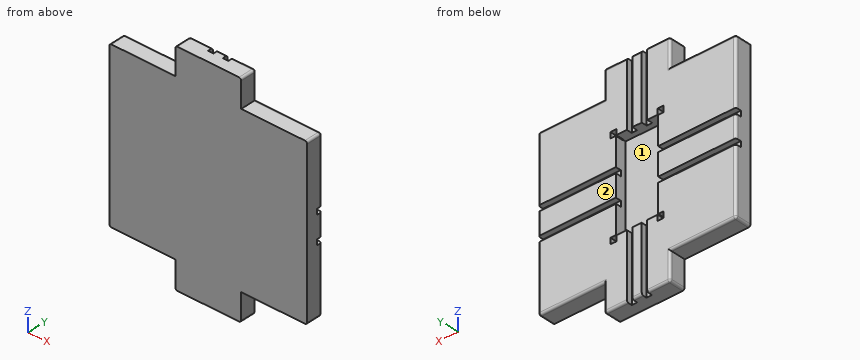
```python
from build123d import *

# Parameters (mm, degrees)
SKETCH1_W                                  = 180
SKETCH1_H                                  = 150
BOSS_EXTRUDE1_DEPTH                        = 15
SKETCH7_W                                  = 60
SKETCH7_H                                  = 25
BOSS_EXTRUDE6_DEPTH                        = 15
FILLET1_R                                  = 2
SKETCH2_W                                  = 38.5
SKETCH2_H                                  = 82
CUT_EXTRUDE1_DEPTH                         = 10
CUT_EXTRUDE3_DEPTH                         = 5
SKETCH11_W                                 = 5.5
SKETCH11_H                                 = 5.5
CUT_EXTRUDE6_DEPTH                         = 7
MIRROR3_AT_THE_SECOND_PLANE_COPY_1_SKETC_W = 5.5
MIRROR3_AT_THE_SECOND_PLANE_COPY_1_SKETC_H = 5.5
MIRROR3_AT_THE_SECOND_PLANE_COPY_1_DEPTH   = 7
MIRROR4_AT_THE_SECOND_PLANE_COPY_1_DEPTH   = 5


with BuildPart() as part:
    # Sketch1 → Boss-Extrude1 (new body)
    with BuildSketch(Plane(origin=(0, 0, 0), x_dir=(1, 0, 0), z_dir=(0, 1, 0))):
        Rectangle(SKETCH1_W, SKETCH1_H)
    extrude(amount=BOSS_EXTRUDE1_DEPTH)

    # Sketch7 → Boss-Extrude6 (add)
    with BuildSketch(Plane(origin=(0, 0, 0), x_dir=(1, 0, 0), z_dir=(0, 1, 0))):
        with Locations((0, -87.5)):
            Rectangle(SKETCH7_W, SKETCH7_H)
        with Locations((0, 87.5)):
            Rectangle(SKETCH7_W, SKETCH7_H)
    extrude(amount=BOSS_EXTRUDE6_DEPTH)

    # Fillet1
    fillet1_edges = [part.edges().sort_by_distance(p)[0] for p in [
        (-90, 15, 0),
        (60, 15, 75),
        (-60, 15, 75),
        (-30, 7.5, 100),
        (30, 7.5, 100),
        (-30, 15, 87.5),
        (0, 15, 100),
        (30, 15, 87.5),
        (-60, 15, -75),
        (0, 15, -100),
        (30, 7.5, -100),
        (-30, 15, -87.5),
        (-30, 7.5, -100),
        (30, 15, -87.5),
        (90, 15, 0),
        (90, 7.5, 75),
        (-90, 7.5, 75),
        (-90, 7.5, -75),
        (90, 7.5, -75),
        (60, 15, -75),
    ]]
    fillet(fillet1_edges, radius=FILLET1_R)

    # Sketch2 → Cut-Extrude1 (cut)
    with BuildSketch(Plane(origin=(0, 15, 0), x_dir=(1, 0, 0), z_dir=(0, 1, 0))):
        Rectangle(SKETCH2_W, SKETCH2_H)
    extrude(amount=-CUT_EXTRUDE1_DEPTH, mode=Mode.SUBTRACT)

    # Sketch10 → Cut-Extrude3 (cut)
    with BuildSketch(Plane(origin=(0, 15, 0), x_dir=(1, 0, 0), z_dir=(0, 1, 0))):
        Polygon((-9.25, -40.5), (-9.25, -33.162899401), (-4.25, -33.162899401), (-4.25, -40.5), (-4.25, -105.687952047), (-9.25, -105.687952047), align=None)
        Polygon((-99.022946063, 15), (-19.25, 15), (-11.555108838, 15), (-11.555108838, 10), (-19.25, 10), (-99.022946063, 10), align=None)
    cut_extrude3 = extrude(amount=-CUT_EXTRUDE3_DEPTH, mode=Mode.SUBTRACT)

    # Sketch11 → Cut-Extrude6 (cut)
    with BuildSketch(Plane(origin=(0, 15, 0), x_dir=(1, 0, 0), z_dir=(0, 1, 0))):
        with Locations((-21.549732367, 43.299732367)):
            Rectangle(SKETCH11_W, SKETCH11_H)
    cut_extrude6 = extrude(amount=-CUT_EXTRUDE6_DEPTH, mode=Mode.SUBTRACT)

    # Mirror3: Cut-Extrude6 across plane
    add(cut_extrude6.mirror(Plane(origin=(0, 0, 0), x_dir=(0, 0, 1), z_dir=(1, 0, 0))), mode=Mode.SUBTRACT)

    # Mirror3 at the second plane: Cut-Extrude6 across plane
    add(cut_extrude6.mirror(Plane.XY), mode=Mode.SUBTRACT)

    # Mirror3 at the second plane copy 1 sketc → Mirror3 at the second plane copy 1 (cut)
    with BuildSketch(Plane(origin=(0, 15, 0), x_dir=(-1, 0, 0), z_dir=(0, 1, 0))):
        with Locations((-21.549732367, 43.299732367)):
            Rectangle(MIRROR3_AT_THE_SECOND_PLANE_COPY_1_SKETC_W, MIRROR3_AT_THE_SECOND_PLANE_COPY_1_SKETC_H)
    extrude(amount=-MIRROR3_AT_THE_SECOND_PLANE_COPY_1_DEPTH, mode=Mode.SUBTRACT)

    # Mirror4: Cut-Extrude3 across plane
    add(cut_extrude3.mirror(Plane(origin=(0, 0, 0), x_dir=(0, 0, 1), z_dir=(1, 0, 0))), mode=Mode.SUBTRACT)

    # Mirror4 at the second plane: Cut-Extrude3 across plane
    add(cut_extrude3.mirror(Plane.XY), mode=Mode.SUBTRACT)

    # Mirror4 at the second plane copy 1 sketc → Mirror4 at the second plane copy 1 (cut)
    with BuildSketch(Plane(origin=(0, 15, 0), x_dir=(-1, 0, 0), z_dir=(0, 1, 0))):
        Polygon((-9.25, -40.5), (-9.25, -33.162899401), (-4.25, -33.162899401), (-4.25, -40.5), (-4.25, -105.687952047), (-9.25, -105.687952047), align=None)
        Polygon((-99.022946063, 15), (-19.25, 15), (-11.555108838, 15), (-11.555108838, 10), (-19.25, 10), (-99.022946063, 10), align=None)
    extrude(amount=-MIRROR4_AT_THE_SECOND_PLANE_COPY_1_DEPTH, mode=Mode.SUBTRACT)


solid = part.part
```
For this review, take the finished solid that the model builds, in its own axes (mm). Face numbers are marked on the shaded views. Coordinates: 2 decimals unless noted, no trailing zeros. Write each loop counter-clockwise with the first axis right and the second up, starting at its lowest first coordinate (ties: lowest second). Pieces come first, ordered by that corner, then holes. Notation, with made-up numbers: (3.5, 70) - (7.5, 70) arc R15 ccw to (7.5, 76) - close; hole circle Ø8 at (-25.75, 69). An arc over 180 degrees is marked (long way). Put each result on its own line as item: value.
1. Add section D-D, the plane z = -25. Give the boundary of the cut face in (x, y).
Values found:
outline: (-90, 0) - (90, 0) - (90, 13) arc R2 ccw to (88, 15) - (19.25, 15) - (19.25, 5) - (-19.25, 5) - (-19.25, 15) - (-88, 15) arc R2 ccw to (-90, 13) - close
2. Add section B-B, the plane x = 68. Give the boundary of the cut face in (y, z).
Values found:
outline: (0, -75) - (13, -75) arc R2 ccw to (15, -73) - (15, -15) - (10, -15) - (10, -10) - (15, -10) - (15, 10) - (10, 10) - (10, 15) - (15, 15) - (15, 73) arc R2 ccw to (13, 75) - (0, 75) - close
3. Add section C-C, the plane x = -7. Give the boundary of the cut face in (y, z), then the cut area to 3 significant figures.
Values found:
outline: (0, -100) - (10, -100) - (10, -41) - (5, -41) - (5, 41) - (10, 41) - (10, 100) - (0, 100) - close
area: 1,590 mm²
4. Wall thickness on probe 1 along Z at (x, y) = (67.5, 11.5); probe 2 along X at (y, z) = (13.25, 39.5); probe 3 along Z at (x, y) = (23, 14.5): over which ranges is each line inside the solid? List them lowest first.
Values found:
probe 1: -75 to -15, -10 to 10, 15 to 75
probe 2: -89.98 to -19.25, 19.25 to 89.98
probe 3: -99.32 to -46.05, -40.55 to -15, -10 to 10, 15 to 40.55, 46.05 to 99.32
5. Add section A-A, the plane z = 82. Give the boundary of the cut face in (x, y).
Values found:
outline: (-30, 0) - (30, 0) - (30, 13) arc R2 ccw to (28, 15) - (9.25, 15) - (9.25, 10) - (4.25, 10) - (4.25, 15) - (-4.25, 15) - (-4.25, 10) - (-9.25, 10) - (-9.25, 15) - (-28, 15) arc R2 ccw to (-30, 13) - close
6. For pin 1 (4 mm diameter, centred on x = 54.5, y = 13.5, fed in from -Z); pin 2 (1.5 mm diameter, centred on x = 6, z = -62, fed in from +Y); pin 3 (4 mm diameter, centred on y = 5.5, z = -86.5, fed in from +X), all flat-tipped, find the tip position at first contact; note any pin that passes through.
Values found:
pin 1: z = -75
pin 2: y = 10
pin 3: x = 30
7. Mouldability with a two-part tool opening along X and no side actions: class the marked faces 1 and 2 as released by +X, released by -X, zero draft, split by the parting line, or undercut.
Values found:
face 1: undercut
face 2: zero draft
